Geometry check sheet. Reference: the model listing, model coordinates, mm. Face numbers are marked on the shaded views. Round coordinates to 2 decimals unless told otherwise and drop trailing zeros. Order: outer loops, then holes, each group sorted by start corner. A loop starts at its lowest first (then second) coordinate and runs counter-clockwise, first axis right, second up. Notation, with made-up numbers: (48.5, 53.25) - (70.5, 53.25) arc R9 ccw to (70.5, 57.25) - close; hole circle Ø7 at (59.5, 81.5). An arc over 180 degrees is marked (long way). One line per question, with ' | ' between items. Start each with the question number.
Q1. Sectioned sample at C-C, the plane y = -32.5. Enter the section's corners in (x, z).
Q2. Sectioned sample at D-D, the plane z = -11. Enter the section's corners in (x, y), then the cut area to 3 significant figures.
Q3. Sectioned sample at A-A, the plane z = 28. Enter the section's corners in (x, y), then the cut area to 3 significant figures.
Q4. Sectioned sample at B-B, the plane x = -499. Enter the section's corners in (y, z), then the cut area to 3 significant figures.
Q5. Gauge pin test, flat ends, axial feed: P1, Ø4, axis at x = -468.5, z = 33, coming from the +Y side; P2, Ø8, axis at y = -16, z = 75, coming from the -X side; P3, Ø3, axis at x = -527, y = -22, coming from the +Z side; P4, Ø12, axis at x = -573.5, y = -44.5, coming from the +Z side. Record the tip position at first contact, or that the pin passes through.
Q6. Material ranges on line 1 along X through (y, z) = (-24, 18); line 2 along X through (y, z) = (-39, 40.5); line 3 along Z through (x, y) = (-534.5, -32.5), recorded low to high.
Q7. Mould release check, pull along X, two halves, no side actions. Record for the marked faces 1, 2 and 3: +X half, -X half, draft (parallel to the pull), parting line (faces both ways), or undercut.
```python
from build123d import *

# Parameters (mm, degrees)
F0_R     = 32.5
F1_DEPTH = 50


with BuildPart() as f1:
    # F0 (on Front) → F1 (new body)
    with BuildSketch(Plane.XZ):
        with BuildLine():
            Line((-395.797376, 46.109863), (-395.797376, 121.109863))
            Line((-395.797376, 121.109863), (-520.797376, 121.109863))
            ThreePointArc((-520.797376, 121.109863), (-573.830384, 99.142871), (-595.797376, 46.109863))
            ThreePointArc((-595.797376, 46.109863), (-573.830384, -6.923146), (-520.797376, -28.890137))
            Line((-520.797376, -28.890137), (-395.797376, -28.890137))
            Line((-395.797376, -28.890137), (-395.797376, 46.109863))
        make_face()
        with Locations((-520.797376, 46.109863)):
            Circle(F0_R, mode=Mode.SUBTRACT)
    extrude(amount=F1_DEPTH)


solid = f1.part
```
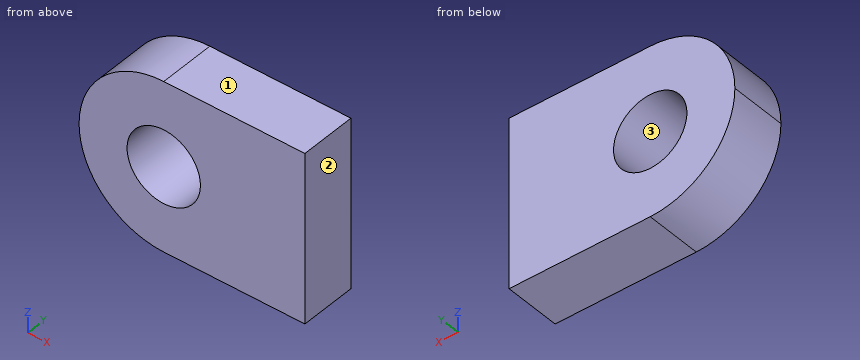
Determined:
1) outline: (-595.8, 46.11) arc R75 ccw to (-520.8, -28.89) - (-395.8, -28.89) - (-395.8, 121.11) - (-520.8, 121.11) arc R75 ccw to start; hole circle Ø65 at (-520.8, 46.11)
2) outline: (-569.41, -50) - (-395.8, -50) - (-395.8, 0) - (-569.41, 0) - close | area: 8,680 mm2
3) outline: (-593.58, -50) - (-547.78, -50) - (-547.78, 0) - (-593.58, 0) - close; (-493.81, -50) - (-395.8, -50) - (-395.8, 0) - (-493.81, 0) - close | area: 7,190 mm2
4) outline: (-50, -28.89) - (0, -28.89) - (0, 22) - (-50, 22) - close; (-50, 70.22) - (0, 70.22) - (0, 121.11) - (-50, 121.11) - close | area: 5,090 mm2
5) P1: stops at y = 0 | P2: stops at x = -591.55 | P3: stops at z = 120.96 | P4: stops at z = 104.79
6) line 1: x = -590.33 to -537.11, -504.49 to -395.8 | line 2: x = -595.59 to -552.81, -488.79 to -395.8 | line 3: z = -27.63 to 16.64, 75.58 to 119.85
7) face 1: draft | face 2: +X half | face 3: undercut
